Here's how the part is built. I have some questions about the finished solid (model axes, mm). Face numbers are marked on the shaded views. A direction names the side the tool comes from. Round coordinates to 2 decimals unless told otherwise and drop trailing zeros. Loops run counter-clockwise (first coordinate to the right, second up) from the corner with the lowest first, then second, coordinate; pieces in that order, holes last. Notation, with made-up numbers: (87, 86.25) -> (120, 86.25) arc R32 ccw to (120, 117.25) -> close; hole circle Ø3 at (32.5, 57.25). An arc over 180 degrees is marked (long way). Use CSV: the item, a comma, the result in double quotes. Start each with the question number.
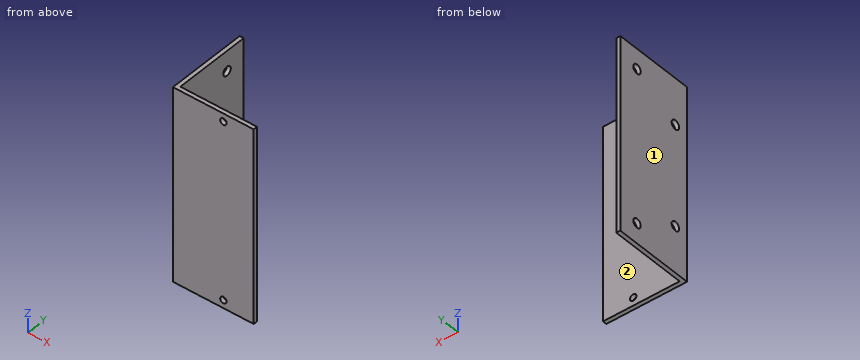
from build123d import *

# Parameters (mm, degrees)
EXTRUDE_1_DEPTH     = 96
SKETCH_2_R          = 1.6
CUT_EXTRUDE_1_DEPTH = 41
SKETCH_3_R          = 2.25
CUT_EXTRUDE_2_DEPTH = 41


with BuildPart() as part:
    # Эскиз1 → Бобышка-Вытянуть1 (new body)
    with BuildSketch(Plane.XY):
        Polygon((0, 0), (40, 0), (40, 2), (2, 2), (2, 40), (0, 40), align=None)
    extrude(amount=EXTRUDE_1_DEPTH)

    # Эскиз2 → Вырез-Вытянуть1 (cut, through all)
    with BuildSketch(Plane.XZ):
        with Locations((25, 92)):
            Circle(SKETCH_2_R)
        with Locations((25, 4)):
            Circle(SKETCH_2_R)
    extrude(amount=-CUT_EXTRUDE_1_DEPTH, mode=Mode.SUBTRACT)

    # Эскиз3 → Вырез-Вытянуть2 (cut, through all)
    with BuildSketch(Plane.ZY):
        with Locations((10, 30)):
            Circle(SKETCH_3_R)
        with Locations((86, 30)):
            Circle(SKETCH_3_R)
        with Locations((73, 7)):
            Circle(SKETCH_3_R)
        with Locations((23, 7)):
            Circle(SKETCH_3_R)
    extrude(amount=-CUT_EXTRUDE_2_DEPTH, mode=Mode.SUBTRACT)


solid = part.part
Q1. I want a section at B-B, the plane z = 86. List the corners of the cut face in (x, y) for me, then the cut area to 3 significant figures.
Q2. I need wall thicknesses on line 1 along X through (y, z) = (1.6, 92); line 2 along Y through (x, z) = (0.7, 73); line 3 along Y through (x, z) = (16, 61). Which ranges of each line are inside material? Lowest first, please.
Q3. For the marked faces 1 and 2, which set-ups out of +Z, -Z, +X, -X, +Y, -Y let a thin tool reach every point of the face, with its end or its side?
Q4. I want a section at D-D, the plane z = 4. List the corners of the cut face in (x, y) for me.
Q5. I want a section at C-C, the plane z = 66.5. List the corners of the cut face in (x, y) for me, then the cut area to 3 significant figures.
Q6. I want a section at A-A, the plane y = 7. List the corners of the cut face in (x, z) for me, then the cut area to 3 significant figures.
Q7. Will these pins go through, and if not, where does the flat tip stop? pin 1 Ø2 at (y, z) = (11.5, 14.5) entering from +X; pin 2 Ø19 at (x, z) = (14, 54.5) entering from +Y.
Values found:
1,outline,"(0, 0) -> (40, 0) -> (40, 2) -> (2, 2) -> (2, 27.75) -> (0, 27.75) -> close; (0, 32.25) -> (2, 32.25) -> (2, 40) -> (0, 40) -> close"
1,area,"147 mm2"
2,line 1,"0 to 23.4, 26.6 to 40"
2,line 2,"0 to 4.75, 9.25 to 40"
2,line 3,"0 to 2"
3,face 1,"+Z, -Z, -X, +Y, -Y"
3,face 2,"+Z, -Z, +X, +Y"
4,outline,"(0, 0) -> (23.4, 0) -> (23.4, 2) -> (2, 2) -> (2, 40) -> (0, 40) -> close; (26.6, 0) -> (40, 0) -> (40, 2) -> (26.6, 2) -> close"
5,outline,"(0, 0) -> (40, 0) -> (40, 2) -> (2, 2) -> (2, 40) -> (0, 40) -> close"
5,area,"156 mm2"
6,outline,"(0, 0) -> (2, 0) -> (2, 20.75) -> (0, 20.75) -> close; (0, 25.25) -> (2, 25.25) -> (2, 70.75) -> (0, 70.75) -> close; (0, 75.25) -> (2, 75.25) -> (2, 96) -> (0, 96) -> close"
6,area,"174 mm2"
7,pin 1,"x = 2"
7,pin 2,"y = 2"
